from build123d import *

# Parameters (mm, degrees)
SKETCH2_R          = 1.5
BOSS_EXTRU_1_DEPTH = 1
ESQUISSE1_W        = 5
ESQUISSE1_H        = 3.690231621


with BuildPart() as part:
    # Sketch2 → Boss.-Extru.1 (new body)
    with BuildSketch(Plane(origin=(0, 0, 0), x_dir=(1, 0, 0), z_dir=(0, 1, 0))):
        with BuildLine():
            Line((-4.607142857, 6.843736895), (-11.230519481, 2.384938615))
            ThreePointArc((-11.230519481, 2.384938615), (-12.5, 0), (-11.230519481, -2.384938615))
            Line((-11.230519481, -2.384938615), (-4.607142857, -6.843736895))
            ThreePointArc((-4.607142857, -6.843736895), (0, -8.25), (4.607142857, -6.843736895))
            Line((4.607142857, -6.843736895), (11.230519481, -2.384938615))
            ThreePointArc((11.230519481, -2.384938615), (12.5, 0), (11.230519481, 2.384938615))
            Line((11.230519481, 2.384938615), (4.607142857, 6.843736895))
            ThreePointArc((4.607142857, 6.843736895), (0, 8.25), (-4.607142857, 6.843736895))
        make_face()
        with Locations(Location((-9.625, 0, 0), (0, 0, 270))):
            Circle(SKETCH2_R, mode=Mode.SUBTRACT)
        with Locations(Location((9.625, 0, 0), (0, 0, 270))):
            Circle(SKETCH2_R, mode=Mode.SUBTRACT)
    extrude(amount=BOSS_EXTRU_1_DEPTH)

    # Esquisse1 → Révolution1 (revolve)
    with BuildSketch(Plane.XY, mode=Mode.PRIVATE) as r_volution1_sk:
        with BuildLine():
            ThreePointArc((0, 10), (-2.136216237, 8.92264844), (-2.996693627, 6.690231621))
            Line((-2.996693627, 6.690231621), (0, 6.690231621))
            Line((0, 6.690231621), (0, 10))
        make_face()
        with BuildLine():
            ThreePointArc((-2.996693627, 6.690231621), (-4.413044266, 6.105614645), (-5, 4.690231621))
            Line((-5, 4.690231621), (0, 4.690231621))
            Line((0, 4.690231621), (0, 6.690231621))
            Line((0, 6.690231621), (-2.996693627, 6.690231621))
        make_face()
        with Locations((-2.5, 2.845115811)):
            Rectangle(ESQUISSE1_W, ESQUISSE1_H)
    revolve(r_volution1_sk.sketch.rotate(Axis((0, -1.148221133, 0), (0, 1, 0)), 270), axis=Axis((0, -1.148221133, 0), (0, 1, 0)))


solid = part.part
Can you work these out from the model? Positions are in its coordinate system, mm. A direction names the side the tool comes from. Coordinates: 2 decimals unless noted, no trailing zeros. Write each loop counter-clockwise with the first axis right and the second up, starting at its lowest first coordinate (ties: lowest second). Pieces come first, ordered by that corner, then holes. Notation, with made-up numbers: M 72,28.25 L 78,28.25 A29 ccw 78,61.25 Z; hole C -18.5,6 d8. An arc over 180 degrees is marked long. Use one line per item in the form item = value.
Q1. For faces 5 (the flat face through (-6, 1, 0)), 6 (the cylindrical face through (0.07, 0.49, -8.25)), which set-ups out of +Z, -Z, +X, -X, +Y, -Y let a thin tool reach every point of the face, with its end or its side?
Model answer:
face_5 = +Y
face_6 = -Z, +Y, -Y
Q2. We'd pull the mould along X, two halves only. Please class faces 1 (the cylindrical face through (8.16, 0.49, -0.33)), 2 (the cylindrical face through (-11.09, 0.49, -0.33)), 3 (the flat face through (7.872, 0.493, 4.646)), 4 (the flat face through (-7.872, 0.493, -4.646)): +X half, -X half, draft (parallel to the pull), parting line (faces both ways), or undercut.
Model answer:
face_1 = undercut
face_2 = undercut
face_3 = +X half
face_4 = -X half
Q3. If we section it at D-D (x = -7.5): Write out the boundary of the cut face in (y, z), then the cut area to 3 significant figures.
Model answer:
outline = M 0,-4.9 L 1,-4.9 L 1,4.9 L 0,4.9 Z
area = 9.79 mm^2
Q4. If we section it at A-A (x = 10.5): Write out the boundary of the cut face in (y, z), then the cut area to 3 significant figures.
Model answer:
outline = M 0,-2.88 L 1,-2.88 L 1,-1.22 L 0,-1.22 Z; M 0,1.22 L 1,1.22 L 1,2.88 L 0,2.88 Z
area = 3.32 mm^2
Q5. For P1, Ø3, axis at x = 2, z = -2.5, coming from the +Y side; P2, Ø5, axis at x = 3, z = 4, coming from the +Y side; P3, Ø1, axis at y = 9, z = 0.5, coming from the -X side, each with a flat end and sliding along its axis, tell me the tip position at first contact or that it passes through.
Model answer:
P1 = 9.32
P2 = 8.44
P3 = -2.42
Q6. If we section it at C-C (z = 1): State how many separate pieces and enclosed holes the cut face has, then the cut area to 3 significant figures.
Model answer:
separate_pieces = 3
enclosed_holes = 0
area = 87.6 mm^2
Q7. If we section it at B-B (y = 2.75): Write out the boundary of the cut face in (x, z).
Model answer:
outline = C 0,0 d10
Q8. I need wall thicknesses on line 1 along Y through (x, z) = (-7.25, -4.5); line 2 along Z through (x, y) = (2, 8); line 3 along X through (y, z) = (6, -2). Which ranges of each line are inside material? Lowest first, please. Write a range as from..to.
Model answer:
line_1 = 0..1
line_2 = -1.86..1.86
line_3 = -4.04..4.04
